The model under review builds one solid part; all positions refer to its coordinate system, in mm. A direction names the side the tool comes from. Round coordinates to 2 decimals unless told otherwise and drop trailing zeros. Loops run counter-clockwise (first coordinate to the right, second up) from the corner with the lowest first, then second, coordinate; pieces in that order, holes last. Notation, with made-up numbers: (22.5, 22) -> (70.5, 22) arc R33 cw to (70.5, 60) -> close; hole circle Ø4 at (55, 44.25). An arc over 180 degrees is marked (long way). Use CSV: the item, a comma, the result in double quotes. Start each with the question number.
```python
from build123d import *

# Parameters (mm, degrees)
SKETCH1_W           = 42.3
SKETCH1_H           = 42.3
BOSS_EXTRUDE1_DEPTH = 48
CUT_EXTRUDE1_DEPTH  = 57.556564606
SKETCH2_3_R         = 1.5
CUT_EXTRUDE2_DEPTH  = 4.5
SKETCH2_4_R         = 11
BOSS_EXTRUDE2_DEPTH = 2
SKETCH2_5_R         = 2.5
BOSS_EXTRUDE3_DEPTH = 24


with BuildPart() as part:
    # Sketch1 → Boss-Extrude1 (new body)
    with BuildSketch(Plane(origin=(0, 0, 0), x_dir=(1, 0, 0), z_dir=(0, 1, 0))):
        Rectangle(SKETCH1_W, SKETCH1_H)
    extrude(amount=BOSS_EXTRUDE1_DEPTH)

    # Sketch2 → Cut-Extrude1 (cut, through all)
    with BuildSketch(Plane(origin=(0, 48, 0), x_dir=(1, 0, 0), z_dir=(0, 1, 0))):
        Polygon((-21.15, 21.15), (-21.15, 17.15), (-17.15, 21.15), align=None)
        Polygon((21.15, 21.15), (17.15, 21.15), (21.15, 17.15), align=None)
        Polygon((21.15, -17.15), (17.15, -21.15), (21.15, -21.15), align=None)
        Polygon((-17.15, -21.15), (-21.15, -17.15), (-21.15, -21.15), align=None)
    extrude(amount=-CUT_EXTRUDE1_DEPTH, mode=Mode.SUBTRACT)

    # Sketch2_3 → Cut-Extrude2 (cut)
    with BuildSketch(Plane(origin=(0, 48, 0), x_dir=(1, 0, 0), z_dir=(0, 1, 0))):
        with Locations(Location((15.5, 15.5, 0), (0, 0, 270))):
            Circle(SKETCH2_3_R)
        with Locations(Location((15.5, -15.5, 0), (0, 0, 270))):
            Circle(SKETCH2_3_R)
        with Locations(Location((-15.5, -15.5, 0), (0, 0, 270))):
            Circle(SKETCH2_3_R)
        with Locations(Location((-15.5, 15.5, 0), (0, 0, 270))):
            Circle(SKETCH2_3_R)
    extrude(amount=-CUT_EXTRUDE2_DEPTH, mode=Mode.SUBTRACT)

    # Sketch2_4 → Boss-Extrude2 (add)
    with BuildSketch(Plane(origin=(0, 48, 0), x_dir=(1, 0, 0), z_dir=(0, 1, 0))):
        with Locations(Location((0, 0, 0), (0, 0, 270))):
            Circle(SKETCH2_4_R)
    extrude(amount=BOSS_EXTRUDE2_DEPTH)

    # Sketch2_5 → Boss-Extrude3 (add)
    with BuildSketch(Plane(origin=(0, 48, 0), x_dir=(1, 0, 0), z_dir=(0, 1, 0))):
        with Locations(Location((0, 0, 0), (0, 0, 270))):
            Circle(SKETCH2_5_R)
    extrude(amount=BOSS_EXTRUDE3_DEPTH)


solid = part.part
```
1. Take a section at B-B, the plane y = 41. Give the boundary of the cut face in (x, z).
2. For faces 5 (the face through (16, 43.5, 15)), 6 (the face through (0, 0, 0)), list the 3-axis set-ups (+Z, -Z, +X, -X, +Y, -Y) from which the entire face can be reached by the end or side of a thin tool; tool diameter is ignored.
3. Take a section at A-A, the plane x = -15.5. Give the boundary of the cut face in (y, z).
4. The part is to be moulded in two halves that separate along X. For faces 1 (the face through (-15.43, 45.78, -17)), 2 (the face through (21.15, 24, 0)), 3 (the face through (-19.1, 24.3, 19.2)), 4 (the face through (-2.44, 60.85, -0.54)), say which applies: pulls with the +X half, pulls with the -X half, needs draft (parallel to the pull), parting line crosses it, or undercut.
5. Take a section at C-C, the plane z = -15.5. Give the boundary of the cut face in (x, y), then the cut area to 3 significant figures.
6. Take a section at D-D, the plane y = 60. Give the boundary of the cut face in (x, z), then the cut area to 3 significant figures.
7. Clearance check with flat-ended pins moving along their axes: P1, Ø3.5, axis at x = -15, z = 16, coming from the +Y side; P2, Ø1.5, axis at x = -15, z = -15, coming from the +Y side; P3, Ø10, axis at x = 8.5, y = 60, coming from the +Z side; P4, Ø10, axis at x = 10, z = 6.5, coming from the +Y side. State where each tip first meets the part, or that it passes through.
8. For line 1 along X through (y, z) = (45.55, -15.5); line 2 along Y through (x, z) = (-3.5, 0); line 3 along Y through (x, z) = (10, 5), list the stretches that pass through material, from the lowest coordinate up. Write a range as from..to.
Results:
1,outline,"(-21.15, -17.15) -> (-17.15, -21.15) -> (17.15, -21.15) -> (21.15, -17.15) -> (21.15, 17.15) -> (17.15, 21.15) -> (-17.15, 21.15) -> (-21.15, 17.15) -> close"
2,face 5,"+Y"
2,face 6,"+Z, -Z, +X, -X, -Y"
3,outline,"(0, -21.15) -> (48, -21.15) -> (48, -17) -> (43.5, -17) -> (43.5, -14) -> (48, -14) -> (48, 14) -> (43.5, 14) -> (43.5, 17) -> (48, 17) -> (48, 21.15) -> (0, 21.15) -> close"
4,face 1,"undercut"
4,face 2,"pulls with the +X half"
4,face 3,"pulls with the -X half"
4,face 4,"parting line crosses it"
5,outline,"(-21.15, 0) -> (21.15, 0) -> (21.15, 48) -> (17, 48) -> (17, 43.5) -> (14, 43.5) -> (14, 48) -> (-14, 48) -> (-14, 43.5) -> (-17, 43.5) -> (-17, 48) -> (-21.15, 48) -> close"
5,area,"2,000 mm²"
6,outline,"circle Ø5 at (0, 0)"
6,area,"19.6 mm²"
7,P1,"y = 48"
7,P2,"y = 43.5"
7,P3,"through"
7,P4,"y = 50"
8,line 1,"-21.15..-17, -14..14, 17..21.15"
8,line 2,"0..50"
8,line 3,"0..48"
